from build123d import *

# Parameters (mm, degrees)
F0_W     = 145
F0_H     = 39
F0_R     = 12.5
F1_DEPTH = 3
F2_W     = 60
F2_H     = 30
F3_DEPTH = 17
F4_W     = 7
F4_H     = 5
F5_DEPTH = 2
F6_R     = 2


with BuildPart() as f1:
    # F0 (on Front) → F1 (new body)
    with BuildSketch(Plane.XZ):
        Rectangle(F0_W, F0_H)
        with Locations((-55, 0)):
            Circle(F0_R, mode=Mode.SUBTRACT)
        with Locations((55, 0)):
            Circle(F0_R, mode=Mode.SUBTRACT)
    extrude(amount=F1_DEPTH)

    # F2 (on face) → F3 (join)
    with BuildSketch(Plane.XZ.offset(3)):
        with Locations((0, -4.5)):
            Rectangle(F2_W, F2_H)
    extrude(amount=F3_DEPTH)

    # F4 (on face) → F5 (cut)
    with BuildSketch(Plane.XY.offset(10.5)):
        with Locations((-17.5, -13)):
            Rectangle(F4_W, F4_H)
        with Locations((17.5, -13)):
            Rectangle(F4_W, F4_H)
    extrude(amount=-F5_DEPTH, mode=Mode.SUBTRACT)

    # F6
    f6_edges = [f1.edges().sort_by_distance(p)[0] for p in [
        (0, -3, 10.5),
        (30, -3, -4.5),
        (-30, -3, -4.5),
        (-30, -20, -4.5),
        (0, -20, 10.5),
        (30, -20, -4.5),
    ]]
    fillet(f6_edges, radius=F6_R)


solid = f1.part
Here's how the part is built. I have some questions about the finished solid (model axes, mm). A direction names the side the tool comes from. Coordinates: 2 decimals unless noted, no trailing zeros. Order: outer loops, then holes, each group sorted by start corner. A loop starts at its lowest first (then second) coordinate and runs counter-clockwise, first axis right, second up.
Item 1: If we section it at D-D on z = -16.5: List the corners of the cut face in (x, y) for me.
Result sheet:
outline: (-72.5, -3) - (-32, -3) arc R2 cw to (-30, -5) - (-30, -18) arc R2 ccw to (-28, -20) - (28, -20) arc R2 ccw to (30, -18) - (30, -5) arc R2 cw to (32, -3) - (72.5, -3) - (72.5, 0) - (-72.5, 0) - close
Item 2: For faces 4 (the face through (-30, -11, -5)), 5 (the face through (30, -11, -5)), 6 (the face through (-18, -13, 8.5)), 7 (the face through (0, -11, 10.5)), which set-ups out of +Z, -Z, +X, -X, +Y, -Y let a thin tool reach every point of the face, with its end or its side?
Result sheet:
face 4: +Z, -Z, -X, -Y
face 5: +Z, -Z, +X, -Y
face 6: +Z
face 7: +Z, +X, -X, -Y
Item 3: If we section it at B-B on z = -7.5: List the corners of the cut face in (x, y) for me, plus the area to 4 significant figures.
Result sheet:
outline: (-72.5, -3) - (-65, -3) - (-65, 0) - (-72.5, 0) - close; (-45, -3) - (-32, -3) arc R2 cw to (-30, -5) - (-30, -18) arc R2 ccw to (-28, -20) - (28, -20) arc R2 ccw to (30, -18) - (30, -5) arc R2 cw to (32, -3) - (45, -3) - (45, 0) - (-45, 0) - close; (65, -3) - (72.5, -3) - (72.5, 0) - (65, 0) - close
area: 1,335 mm2
Item 4: For P1, Ø1.6, axis at x = 18, z = 10, coming from the -Y side; P2, Ø1.5, axis at x = 16.5, y = -13, coming from the +Z side; P3, Ø1, axis at y = -13.5, z = 9.5, coming from the -X side; P4, Ø15, axis at x = -55, z = 0, coming from the +Y side, each with a flat end and sliding along its axis, tell me the tip position at first contact or that it passes through.
Result sheet:
P1: stops at y = -19.87
P2: stops at z = 8.5
P3: stops at x = -30
P4: passes through
Item 5: If we section it at C-C on x = -3.5: List the corners of the cut face in (y, z) for me, plus the area to 3 significant figures.
Result sheet:
outline: (-20, -19.5) - (0, -19.5) - (0, 19.5) - (-3, 19.5) - (-3, 12.5) arc R2 cw to (-5, 10.5) - (-18, 10.5) arc R2 ccw to (-20, 8.5) - close
area: 627 mm2
Item 6: If we section it at A-A on x = -55: List the corners of the cut face in (y, z) for me, plus the area to 3 significant figures.
Result sheet:
outline: (-3, -19.5) - (0, -19.5) - (0, -12.5) - (-3, -12.5) - close; (-3, 12.5) - (0, 12.5) - (0, 19.5) - (-3, 19.5) - close
area: 42.0 mm2
Item 7: I need wall thicknesses on line 1 (Z direction, x = -20, y = -6.5); line 2 (Y direction, x = 42.5, z = -9.5); line 3 (X direction, y = -11.5, z = -9). Which ranges of each line are inside material? Lowest first, please.
Result sheet:
line 1: z = -19.5 to 10.5
line 2: y = -3 to 0
line 3: x = -30 to 30
Item 8: If we mould it in two halves opening along Y, with no side actions, what happens to faces 1 (the face through (0, -20, -5)), 2 (the face through (72.5, -1, 0)), 3 (the face through (17, -13, 8.5))? For each: +Y half, -Y half, draft (parallel to the pull), parting line (faces both ways), or undercut.
Result sheet:
face 1: -Y half
face 2: draft
face 3: undercut
